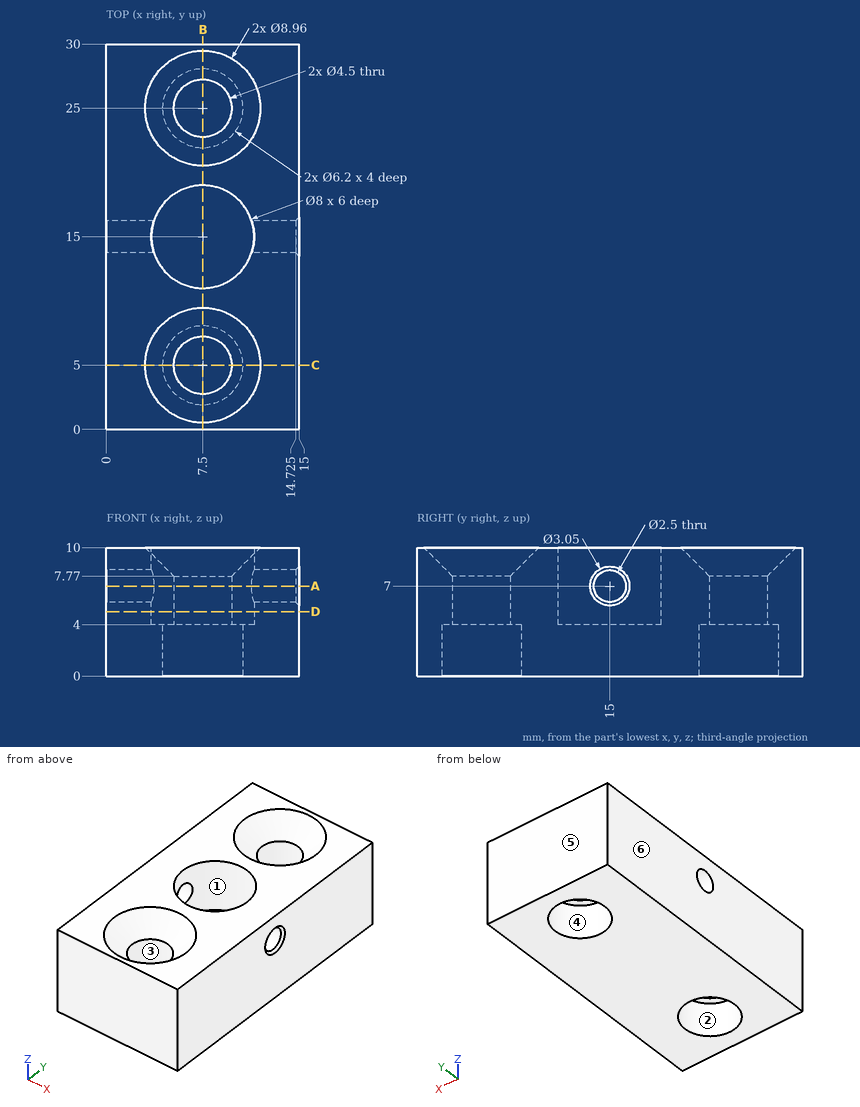
Drawing for the job (mm, zero at the part's lowest x, y, z). A direction names the side the tool comes from. Give positions to 0.01 mm unless a question says otherwise; leave off trailing zeros. Order: outer loops, then holes, each group sorted by start corner. A loop starts at its lowest first (then second) coordinate and runs counter-clockwise, first axis right, second up. Notation, with made-up numbers: M -6.5,35.25 L 11.5,35.25 A11 ccw 11.5,48.25 Z; hole C 85.5,37 d11. An arc over 180 degrees is marked long. Put each result on its own line as item: value. Start each with the question number.
(1) Flat gauge pins, fed straight in: pin 1 Ø5 at (x, y) = (8.5, 24.5) entering from -Z; pin 2 Ø5 at (x, y) = (7.5, 25) entering from -Z; pin 3 Ø1.5 at (x, y) = (8, 13.5) entering from +Z; pin 4 Ø4 at (x, y) = (6.5, 5) entering from +Z. Where does each tip first touch, or does it go through?
(2) Saw through at D-D, the plane z = 5. Write the cut outline in (x, y), then the cut area to 3 significant figures.
(3) Saw through at C-C, the plane y = 5. Write the cut outline in (x, z).
(4) Which spindle directions (+Z, -Z, +X, -X, +Y, -Y) get a long thin tool onto all of the face, cutting with end or side? Do the marked faces 1, 2 and 3. Say none if no direction does.
(5) Mould opens along Y. For the marked faces 4, 5 and 6 say: +Y half, -Y half, draft (parallel to the pull), parting line (faces both ways), or undercut.
(6) Saw through at A-A, the plane z = 7. Write the cut outline in (x, y) (3 decimals).
(7) Saw through at B-B, the plane x = 7.5. Write the cut outline in (y, z), then the cut area to 3 significant figures.
(8) Drill centre lines: line 1 along Y through (x, z) = (7.5, 6.75); line 2 along Y through (x, z) = (7.5, 2.1); line 3 along X through (y, z) = (25, 5). Where is each one in solid material? Low to high.
Check result:
1. pin 1: stops at z = 0
1. pin 2: stops at z = 4
1. pin 3: stops at z = 4
1. pin 4: stops at z = 8.52
2. outline: M 0,0 L 15,0 L 15,30 L 0,30 Z; hole C 7.5,15 d8; hole C 7.5,5 d4.5; hole C 7.5,25 d4.5
2. area: 368 mm2
3. outline: M 0,0 L 4.4,0 L 4.4,4 L 5.25,4 L 5.25,7.77 L 3.02,10 L 0,10 Z; M 9.75,4 L 10.6,4 L 10.6,0 L 15,0 L 15,10 L 11.98,10 L 9.75,7.77 Z
4. face 1: +Z
4. face 2: -Z
4. face 3: +Z, -Z
5. face 4: undercut
5. face 5: +Y half
5. face 6: draft
6. outline: M 0,0 L 15,0 L 15,13.475 L 14.725,13.75 L 11.3,13.75 A4 cw 3.7,13.75 L 0,13.75 Z; M 0,16.25 L 3.7,16.25 A4 cw 11.3,16.25 L 14.725,16.25 L 15,16.525 L 15,30 L 0,30 Z; hole C 7.5,5 d4.5; hole C 7.5,25 d4.5
7. outline: M 0,0 L 1.9,0 L 1.9,4 L 2.75,4 L 2.75,7.77 L 0.52,10 L 0,10 Z; M 7.25,4 L 8.1,4 L 8.1,0 L 21.9,0 L 21.9,4 L 22.75,4 L 22.75,7.77 L 20.52,10 L 19,10 L 19,4 L 11,4 L 11,10 L 9.48,10 L 7.25,7.77 Z; M 27.25,4 L 28.1,4 L 28.1,0 L 30,0 L 30,10 L 29.48,10 L 27.25,7.77 Z
7. area: 138 mm2
8. line 1: y = 0 to 2.75, 7.25 to 11, 19 to 22.75, 27.25 to 30
8. line 2: y = 0 to 1.9, 8.1 to 21.9, 28.1 to 30
8. line 3: x = 0 to 5.25, 9.75 to 15
